from build123d import *

# Parameters (mm, degrees)
BOSS_EXTRUDE1_DEPTH = 20.574
FILLET1_R           = 2.54
FILLET2_R           = 2.54
SKETCH2_R           = 2.667
CUT_EXTRUDE1_DEPTH  = 31.988
SKETCH3_R           = 2.794
CUT_EXTRUDE2_DEPTH  = 31.988


with BuildPart() as part:
    # Sketch1 → Boss-Extrude1 (new body)
    with BuildSketch(Plane.XY):
        Polygon((12.319, 1.5875), (12.319, 29.4005), (15.494, 29.4005), (15.494, -1.5875), (-15.494, -1.5875), (-15.494, 1.5875), align=None)
    extrude(amount=BOSS_EXTRUDE1_DEPTH)

    # Fillet1
    fillet1_edges = [part.edges().sort_by_distance(p)[0] for p in [
        (12.319, 1.5875, 10.287),
    ]]
    fillet(fillet1_edges, radius=FILLET1_R)

    # Fillet2
    fillet2_edges = [part.edges().sort_by_distance(p)[0] for p in [
        (15.494, -1.5875, 10.287),
    ]]
    fillet(fillet2_edges, radius=FILLET2_R)

    # Sketch2 → Cut-Extrude1 (cut, through all)
    with BuildSketch(Plane(origin=(15.494, 0, 0), x_dir=(0, 0, -1), z_dir=(1, 0, 0))):
        with Locations((-10.287, 13.9065)):
            Circle(SKETCH2_R)
    extrude(amount=-CUT_EXTRUDE1_DEPTH, mode=Mode.SUBTRACT)

    # Sketch3 → Cut-Extrude2 (cut, through all)
    with BuildSketch(Plane.XZ.offset(1.5875)):
        with Locations((0, 10.287)):
            Circle(SKETCH3_R)
    extrude(amount=-CUT_EXTRUDE2_DEPTH, mode=Mode.SUBTRACT)


solid = part.part
Read the model definition and answer for the solid it produces. Units are mm, in the model's axes. A direction names the side the tool comes from. Give positions to 0.01 mm unless a question says otherwise; leave off trailing zeros. Loops run counter-clockwise (first coordinate to the right, second up) from the corner with the lowest first, then second, coordinate; pieces in that order, holes last. Notation, with made-up numbers: (58.25, -12.75) - (111.25, -12.75) arc R18 cw to (111.25, -5.75) - close; hole circle Ø5 at (49.5, -33). An arc over 180 degrees is marked (long way). Answer as CSV lines item,"result". Start each with the question number.
1) Find section D-D (x = -5.5). Write down the section's boundary in (y, z), then the cut area to 3 significant figures.
2) Find section B-B (z = 1.75). Write down the section's boundary in (x, y).
3) Which of the six approach directions +Z, -Z, +X, -X, +Y, -Y give full straight-line access (tool end or side, diameter ignored) to faces 4 (the face through (-4, -1.588, 10)), 5 (the face through (-3, 1.588, 10))?
4) Find section A-A (x = 0). Write down the section's boundary in (y, z), then the cut area to 3 significant figures.
5) Find section C-C (z = 11). Write down the section's boundary in (x, y).
6) Each of these flat-tipped pins is pushed along its axis until it touches: pin 1 Ø1 at (y, z) = (4.5, 12) entering from -X; pin 2 Ø2 at (x, z) = (0, 17.5) entering from +Y. Where does it stop, or does it pass through?
7) Straight lines are drawn through the part: L1, parallel to X at y = 7, z = 4.5; L2, parallel to Y at x = 5.5, z = 4.75; L3, parallel to X at y = 0, z = 12.75. For each, find the intervals that lie inside material, in ascending order. Write a range as from..to.
8) Determine the mould class of faces 1 (the face through (13.93, 16.55, 10.63)), 2 (the face through (11.595, 2.351, 10.431)), 3 (the face through (-0.364, -0.022, 13.057)) for opening direction X: released by +X, released by -X, zero draft, split by the parting line, or undercut.
Findings below:
1,outline,"(-1.59, 0) - (1.59, 0) - (1.59, 20.57) - (-1.59, 20.57) - close"
1,area,"65.3 mm^2"
2,outline,"(-15.49, -1.59) - (12.95, -1.59) arc R2.54 ccw to (15.49, 0.95) - (15.49, 29.4) - (12.32, 29.4) - (12.32, 4.13) arc R2.54 cw to (9.78, 1.59) - (-15.49, 1.59) - close"
3,face 4,"+Z, -Z, +X, -X, -Y"
3,face 5,"+Z, -Z, -X, +Y"
4,outline,"(-1.59, 0) - (1.59, 0) - (1.59, 7.49) - (-1.59, 7.49) - close; (-1.59, 13.08) - (1.59, 13.08) - (1.59, 20.57) - (-1.59, 20.57) - close"
4,area,"47.6 mm^2"
5,outline,"(-15.49, -1.59) - (-2.7, -1.59) - (-2.7, 1.59) - (-15.49, 1.59) - close; (2.7, -1.59) - (12.95, -1.59) arc R2.54 ccw to (15.49, 0.95) - (15.49, 11.34) - (12.32, 11.34) - (12.32, 4.13) arc R2.54 cw to (9.78, 1.59) - (2.7, 1.59) - close; (12.32, 16.48) - (15.49, 16.48) - (15.49, 29.4) - (12.32, 29.4) - close"
6,pin 1,"x = 12.32"
6,pin 2,"y = 1.59"
7,L1,"12.32..15.49"
7,L2,"-1.59..1.59"
7,L3,"-15.49..-1.32, 1.32..15.31"
8,face 1,"zero draft"
8,face 2,"released by -X"
8,face 3,"undercut"
